For this review, use the dimensioned drawing (mm, ordinates from the lowest corner) and the shaded views. Coordinates: 2 decimals unless noted, no trailing zeros. Write each loop counter-clockwise with the first axis right and the second up, starting at its lowest first coordinate (ties: lowest second). Pieces come first, ordered by that corner, then holes. Notation, with made-up numbers: M 49.25,30.5 L 79.25,30.5 A10 ccw 79.25,35.5 Z; hole C 45.5,-13.75 d6. An arc over 180 degrees is marked long. One line per question, with ' | ' between items.
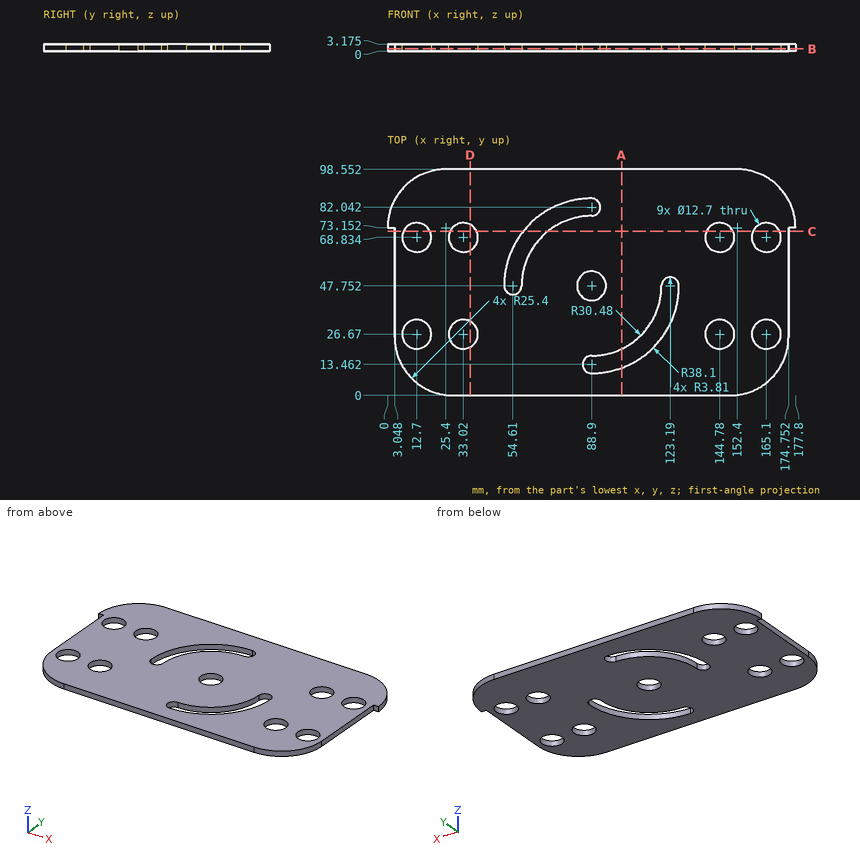
1) We need section A-A on x = 102. State the section outline as (y, z) points (3 decimals).
Responses:
outline: M 0,0 L 11.975,0 L 11.975,3.175 L 0,3.175 Z; M 20.231,0 L 98.552,0 L 98.552,3.175 L 20.231,3.175 Z
2) We need section B-B on z = 1.05. State how many separate pieces and enclosed holes the cut face has, then the cut area to 3 significant figures.
Responses:
separate pieces: 1 | enclosed holes: 11 | area: 14,500 mm^2
3) We need section D-D on x = 36. State the section outline as (y, z) points (3 decimals).
Responses:
outline: M 0,0 L 21.063,0 L 21.063,3.175 L 0,3.175 Z; M 32.277,0 L 63.227,0 L 63.227,3.175 L 32.277,3.175 Z; M 74.441,0 L 98.552,0 L 98.552,3.175 L 74.441,3.175 Z
4) Insertion check: pin 1 Ø10 at (x, y) = (165.1, 26.67) entering from +Z; pin 2 Ø1 at (y, z) = (53, 1) entering from +X; pin 3 Ø1.5 at (x, z) = (176.5, 1.5) entering from -Y; pin 4 Ø1 at (y, z) = (50, 1.5) entering from -X. Each pin has a flat end and moves straight along its axis. Give the tip position at first contact, or say it passes through.
Responses:
pin 1: through | pin 2: x = 174.75 | pin 3: y = 73.15 | pin 4: x = 3.05
5) To check wall thickness, follow line 1 along X through (y, z) = (22.5, 0.9); line 2 along X through (y, z) = (44.5, 2.7); line 3 along Y through (x, z) = (12.7, 2.5). State the ranges of each line that lie inside material, in increasing order. Write a range as [from, to].
Responses:
line 1: [3.21, 7.91], [17.49, 28.23], [37.81, 105.97], [117.43, 139.99], [149.57, 160.31], [169.89, 174.59] | line 2: [3.05, 52.62], [56.6, 83.45], [94.35, 119.21], [126.86, 174.75] | line 3: [5.47, 20.32], [33.02, 62.48], [75.18, 95.15]
6) We need section C-C on y = 71.5. State the section outline as (x, z) points (3 decimals).
Responses:
outline: M 3.048,0 L 6.937,0 L 6.937,3.175 L 3.048,3.175 Z; M 18.463,0 L 27.257,0 L 27.257,3.175 L 18.463,3.175 Z; M 38.783,0 L 59.107,0 L 59.107,3.175 L 38.783,3.175 Z; M 69.793,0 L 139.017,0 L 139.017,3.175 L 69.793,3.175 Z; M 150.543,0 L 159.337,0 L 159.337,3.175 L 150.543,3.175 Z; M 170.863,0 L 174.752,0 L 174.752,3.175 L 170.863,3.175 Z
